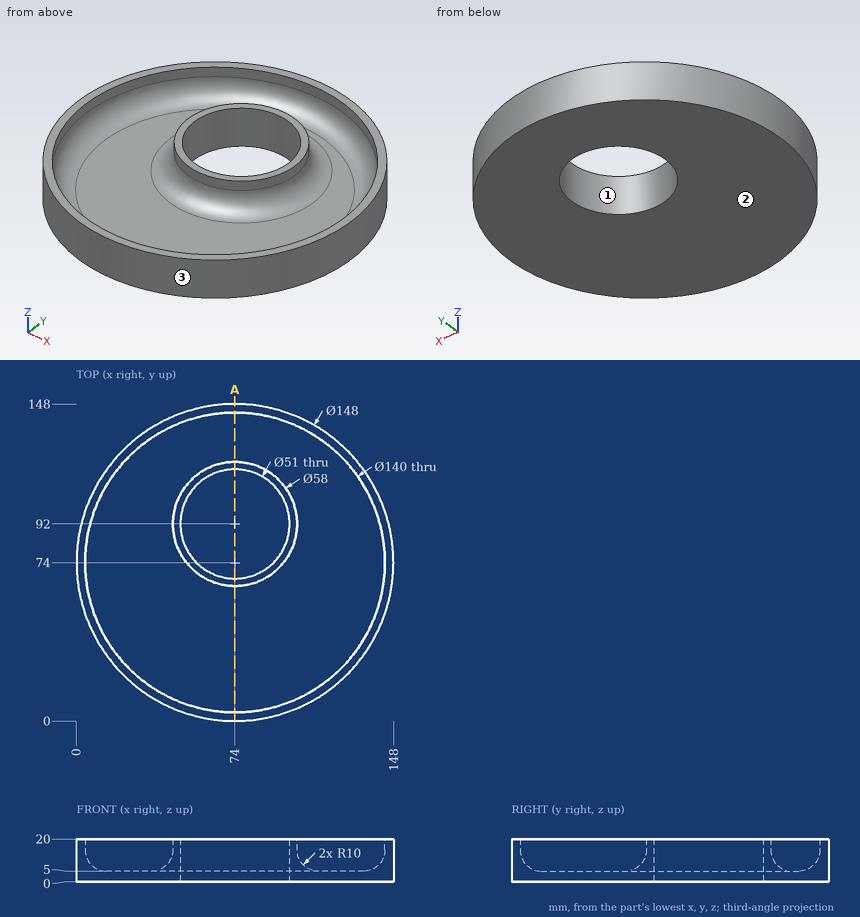
Here's the drawing with two shaded views (mm, measured from the low corner). I have some questions. Round coordinates to 2 decimals unless told otherwise and drop trailing zeros. Loops run counter-clockwise (first coordinate to the right, second up) from the corner with the lowest first, then second, coordinate; pieces in that order, holes last. Notation, with made-up numbers: M 2.25,-6 L 32.25,-6 A23 cw 32.25,22 Z; hole C 50,43 d3. An arc over 180 degrees is marked long. Answer as a JSON object with one key per item and string values. Group by question number.
Q1. Imagine slicing it at A-A, the plane x = 74. Please give me the cut outline in (y, z), then the cut area to 3 significant figures.
Q2. Will these pins go through, and if not, where does the flat tip stop? pin 1 (1 mm diameter, centred on x = 102.5, y = 79, fed in from +Z); pin 2 (1.5 mm diameter, centred on x = 110, z = 17.5, fed in from -Y); pin 3 (1 mm diameter, centred on x = 60.5, y = 64, fed in from +Z).
Q3. Please list where these lines run through material, in increasing order: L1, parallel to Y at x = 74, z = 18.55; L2, parallel to Y at x = 58.5, z = 11.25; L3, parallel to Z at x = 67, y = 48.5.
Q4. We'd pull the mould along X, two halves only. Please class the marked faces 1, 2 and 3: +X half, -X half, draft (parallel to the pull), parting line (faces both ways), or undercut.
Findings:
{
 "1": {"outline": "M 0,0 L 66.5,0 L 66.5,20 L 63,20 L 63,15 A10 cw 53,5 L 14,5 A10 cw 4,15 L 4,20 L 0,20 Z; M 117.5,0 L 148,0 L 148,20 L 144,20 L 144,15 A10 cw 134,5 L 131,5 A10 cw 121,15 L 121,20 L 117.5,20 Z", "area": "796 mm2"},
 "2": {"pin 1": "stops at z = 9.24", "pin 2": "stops at y = 8.94", "pin 3": "stops at z = 9.6"},
 "3": {"L1": "y = 0 to 4, 63 to 66.5, 117.5 to 121, 144 to 148", "L2": "y = 1.64 to 6.49, 66.63 to 71.75, 112.25 to 117.37, 141.51 to 146.36", "L3": "z = 0 to 5"},
 "4": {"face 1": "undercut", "face 2": "draft", "face 3": "parting line"}
}
